```python
from build123d import *

# Parameters (mm, degrees)
BOSS_EXTRUDE1_DEPTH = 8
SKETCH15_W          = 8
SKETCH15_H          = 23.2
BOSS_EXTRUDE2_DEPTH = 15.75
CUT_EXTRUDE2_DEPTH  = 3.1
CUT_EXTRUDE4_DEPTH  = 3.1
CUT_EXTRUDE6_DEPTH  = 3.1
CUT_EXTRUDE7_DEPTH  = 3.1
CUT_EXTRUDE12_DEPTH = 9
SKETCH18_W          = 6.35
SKETCH18_H          = 23.2
BOSS_EXTRUDE3_DEPTH = 12.7


with BuildPart() as part:
    # Sketch1 → Boss-Extrude1 (new body)
    with BuildSketch(Plane.XY.offset(4)):
        with BuildLine():
            Line((-3.6, 0), (-3.6, -16))
            ThreePointArc((-3.6, -16), (0, -19.6), (3.6, -16))
            Line((3.6, -16), (3.6, 0))
            ThreePointArc((3.6, 0), (0, 3.6), (-3.6, 0))
        make_face()
    extrude(amount=-BOSS_EXTRUDE1_DEPTH)

    # Sketch15 → Boss-Extrude2 (add)
    with BuildSketch(Plane.ZY):
        with Locations((0, -8)):
            Rectangle(SKETCH15_W, SKETCH15_H)
    extrude(amount=BOSS_EXTRUDE2_DEPTH)

    # Sketch3 → Cut-Extrude2 (cut)
    with BuildSketch(Plane.XY.offset(4)):
        with BuildLine():
            Line((2.8, -4.8), (2.8, -3.2))
            ThreePointArc((2.8, -3.2), (2.578885438, -2.842229124), (2.16, -2.88))
            ThreePointArc((2.16, -2.88), (0, -3.6), (-2.16, -2.88))
            ThreePointArc((-2.16, -2.88), (-2.578885438, -2.842229124), (-2.8, -3.2))
            Line((-2.8, -3.2), (-2.8, -4.8))
            ThreePointArc((-2.8, -4.8), (-2.578885438, -5.157770876), (-2.16, -5.12))
            ThreePointArc((-2.16, -5.12), (0, -4.4), (2.16, -5.12))
            ThreePointArc((2.16, -5.12), (2.578885438, -5.157770876), (2.8, -4.8))
        make_face()
    extrude(amount=-CUT_EXTRUDE2_DEPTH, mode=Mode.SUBTRACT)

    # Sketch5 → Cut-Extrude4 (cut)
    with BuildSketch(Plane.XY.offset(4)):
        with BuildLine():
            Line((2.8, -12.8), (2.8, -11.2))
            ThreePointArc((2.8, -11.2), (2.578885438, -10.842229124), (2.16, -10.88))
            ThreePointArc((2.16, -10.88), (0, -11.6), (-2.16, -10.88))
            ThreePointArc((-2.16, -10.88), (-2.578885438, -10.842229124), (-2.8, -11.2))
            Line((-2.8, -11.2), (-2.8, -12.8))
            ThreePointArc((-2.8, -12.8), (-2.578885438, -13.157770876), (-2.16, -13.12))
            ThreePointArc((-2.16, -13.12), (0, -12.4), (2.16, -13.12))
            ThreePointArc((2.16, -13.12), (2.578885438, -13.157770876), (2.8, -12.8))
        make_face()
    extrude(amount=-CUT_EXTRUDE4_DEPTH, mode=Mode.SUBTRACT)

    # Sketch7 → Cut-Extrude6 (cut)
    with BuildSketch(Plane(origin=(0, 0, -4), x_dir=(-1, 0, 0), z_dir=(0, 0, -1))):
        with BuildLine():
            Line((2.8, -4.8), (2.8, -3.2))
            ThreePointArc((2.8, -3.2), (2.578885438, -2.842229124), (2.16, -2.88))
            ThreePointArc((2.16, -2.88), (0, -3.6), (-2.16, -2.88))
            ThreePointArc((-2.16, -2.88), (-2.578885438, -2.842229124), (-2.8, -3.2))
            Line((-2.8, -3.2), (-2.8, -4.8))
            ThreePointArc((-2.8, -4.8), (-2.578885438, -5.157770876), (-2.16, -5.12))
            ThreePointArc((-2.16, -5.12), (0, -4.4), (2.16, -5.12))
            ThreePointArc((2.16, -5.12), (2.578885438, -5.157770876), (2.8, -4.8))
        make_face()
    extrude(amount=-CUT_EXTRUDE6_DEPTH, mode=Mode.SUBTRACT)

    # Sketch8 → Cut-Extrude7 (cut)
    with BuildSketch(Plane(origin=(0, 0, -4), x_dir=(-1, 0, 0), z_dir=(0, 0, -1))):
        with BuildLine():
            Line((-2.8, -11.2), (-2.8, -12.8))
            ThreePointArc((-2.8, -12.8), (-2.578885438, -13.157770876), (-2.16, -13.12))
            ThreePointArc((-2.16, -13.12), (0, -12.4), (2.16, -13.12))
            ThreePointArc((2.16, -13.12), (2.578885438, -13.157770876), (2.8, -12.8))
            Line((2.8, -12.8), (2.8, -11.2))
            ThreePointArc((2.8, -11.2), (2.578885438, -10.842229124), (2.16, -10.88))
            ThreePointArc((2.16, -10.88), (0, -11.6), (-2.16, -10.88))
            ThreePointArc((-2.16, -10.88), (-2.578885438, -10.842229124), (-2.8, -11.2))
        make_face()
    extrude(amount=-CUT_EXTRUDE7_DEPTH, mode=Mode.SUBTRACT)

    # Sketch10 → Cut-Revolve1 (revolve, cut)
    with BuildSketch(Plane(origin=(0, -16, 0), x_dir=(1, 0, 0), z_dir=(0, 1, 0))):
        Polygon((3.1, 4), (0, 4), (0, -4), (3.1, -4), (3.1, -3.2), (2.4, -3.2), (2.4, 3.2), (3.1, 3.2), align=None)
    revolve(axis=Axis((0, -16, -4), (0, 0, 1)), mode=Mode.SUBTRACT)

    # Sketch13 → Cut-Revolve4 (revolve, cut)
    with BuildSketch(Plane(origin=(0, 0, 0), x_dir=(1, 0, 0), z_dir=(0, 1, 0))):
        Polygon((3.1, 4), (0, 4), (0, -4), (3.1, -4), (3.1, -3.2), (2.4, -3.2), (2.4, 3.2), (3.1, 3.2), align=None)
    revolve(axis=Axis((0, 0, -4), (0, 0, 1)), mode=Mode.SUBTRACT)

    # Sketch14 → Cut-Extrude12 (cut, through all)
    with BuildSketch(Plane.XY.offset(4)):
        with BuildLine():
            ThreePointArc((-2.26, -8.8), (-2.3972583, -8), (-2.26, -7.2))
            Line((-2.26, -7.2), (-0.8, -7.2))
            Line((-0.8, -7.2), (-0.8, -5.74))
            ThreePointArc((-0.8, -5.74), (0, -5.6027417), (0.8, -5.74))
            Line((0.8, -5.74), (0.8, -7.2))
            Line((0.8, -7.2), (2.26, -7.2))
            ThreePointArc((2.26, -7.2), (2.3972583, -8), (2.26, -8.8))
            Line((2.26, -8.8), (0.8, -8.8))
            Line((0.8, -8.8), (0.8, -10.26))
            ThreePointArc((0.8, -10.26), (0, -10.3972583), (-0.8, -10.26))
            Line((-0.8, -10.26), (-0.8, -8.8))
            Line((-0.8, -8.8), (-2.26, -8.8))
        make_face()
    extrude(amount=-CUT_EXTRUDE12_DEPTH, mode=Mode.SUBTRACT)

    # Sketch18 → Boss-Extrude3 (add, symmetric)
    with BuildSketch(Plane(origin=(0, 0, 0), x_dir=(-1, 0, 0), z_dir=(0, 0, -1))):
        with Locations((12.575, -8)):
            Rectangle(SKETCH18_W, SKETCH18_H)
    extrude(amount=BOSS_EXTRUDE3_DEPTH, both=True)


solid = part.part
```
Input: part model. Units: mm. Frame: model coordinates. A direction names the side the tool comes from. Round coordinates to 2 decimals unless told otherwise and drop trailing zeros. Order: outer loops, then holes, each group sorted by start corner. A loop starts at its lowest first (then second) coordinate and runs counter-clockwise, first axis right, second up. Notation, with made-up numbers: (-22, -32) - (24, -32) arc R29 ccw to (24, -6) - close; hole circle Ø2 at (50.25, 52.25). An arc over 180 degrees is marked (long way). One line per question, with ' | ' between items. Start each with the question number.
1) Ray query, probe 1 along Y at (x, z) = (0, -0.5); probe 2 along Y at (x, z) = (0, 1); probe 3 along Y at (x, z) = (0, -3.6). Return the intervals inside material, ascending.
2) Cut plane D-D, the plane x = -5.75. Return the cut outline in (y, z).
3) Cut plane C-C, the plane y = -17.75. Return the cut outline in (x, z), then the cut area to 3 significant figures.
4) Set-up query: faces 1 (the cylindrical face through (1.43, -2.75, -3.61)), 2 (the cylindrical face through (0, -4.4, 2.5)), 3 (the flat face through (2, -8.8, 0)). Return all of +Z, -Z, +X, -X, +Y, -Y with unobstructed straight access to the full face (end or side cutting, diameter ignored); none if empty.
5) Cut plane A-A, the plane y = -14.25. Return the cut outline in (x, z).
6) Cut plane B-B, the plane z = -2.25. Give the number of separate pieces and of enclosed holes in the cut face, then the cut area to 3 significant figures.
7) Contact query for flat-ended pins moving along their axis: P1, Ø1.2, axis at x = 1.5, z = 0.5, coming from the +Y side; P2, Ø8, axis at x = 0, y = -16, coming from the +Z side; P3, Ø2.5, axis at y = -7, z = 8, coming from the +X side; P4, Ø5, axis at x = -0.5, z = 6, coming from the -Y side. Output: stop coordinate, or through.
8) Pull-direction query (X, two-part tool) for faces 4 (the flat face through (-4, -8, 4)), 5 (the flat face through (-15.75, -8, 0)), 6 (the flat face through (-9.4, -8, 8)), 7 (the cylindrical face through (1.43, -2.75, 3.59)); classes: +X half, -X half, draft (parallel to the pull), parting line (faces both ways), or undercut.
Worked out:
1) probe 1: y = -19.6 to -18.4, -13.6 to -10.4, -5.6 to -2.4, 2.4 to 3.6 | probe 2: y = -19.6 to -18.4, -13.6 to -12.4, -11.6 to -10.4, -5.6 to -4.4, -3.6 to -2.4, 2.4 to 3.6 | probe 3: y = -19.6 to -19.1, -12.9 to -12.4, -11.6 to -10.4, -5.6 to -4.4, -3.6 to -3.1, 3.1 to 3.6
2) outline: (-19.6, -4) - (3.6, -4) - (3.6, 4) - (-19.6, 4) - close
3) outline: (-15.75, -12.7) - (-9.4, -12.7) - (-9.4, -4) - (-2.56, -4) - (-2.56, -3.2) - (-1.64, -3.2) - (-1.64, 3.2) - (-2.56, 3.2) - (-2.56, 4) - (-9.4, 4) - (-9.4, 12.7) - (-15.75, 12.7) - close; (1.64, -3.2) - (2.56, -3.2) - (2.56, -4) - (3.15, -4) - (3.15, 4) - (2.56, 4) - (2.56, 3.2) - (1.64, 3.2) - close | area: 232 mm^2
4) face 1: -Z | face 2: +Z | face 3: +Z, -Z
5) outline: (-15.75, -12.7) - (-9.4, -12.7) - (-9.4, -4) - (-2.56, -4) - (-2.56, -3.2) - (-1.64, -3.2) - (-1.64, 3.2) - (-2.56, 3.2) - (-2.56, 4) - (-9.4, 4) - (-9.4, 12.7) - (-15.75, 12.7) - close; (1.64, -3.2) - (2.56, -3.2) - (2.56, -4) - (3.6, -4) - (3.6, 4) - (2.56, 4) - (2.56, 3.2) - (1.64, 3.2) - close
6) separate pieces: 1 | enclosed holes: 5 | area: 378 mm^2
7) P1: stops at y = 3.49 | P2: stops at z = 4 | P3: stops at x = -9.4 | P4: stops at y = -19.6
8) face 4: draft | face 5: -X half | face 6: +X half | face 7: undercut
